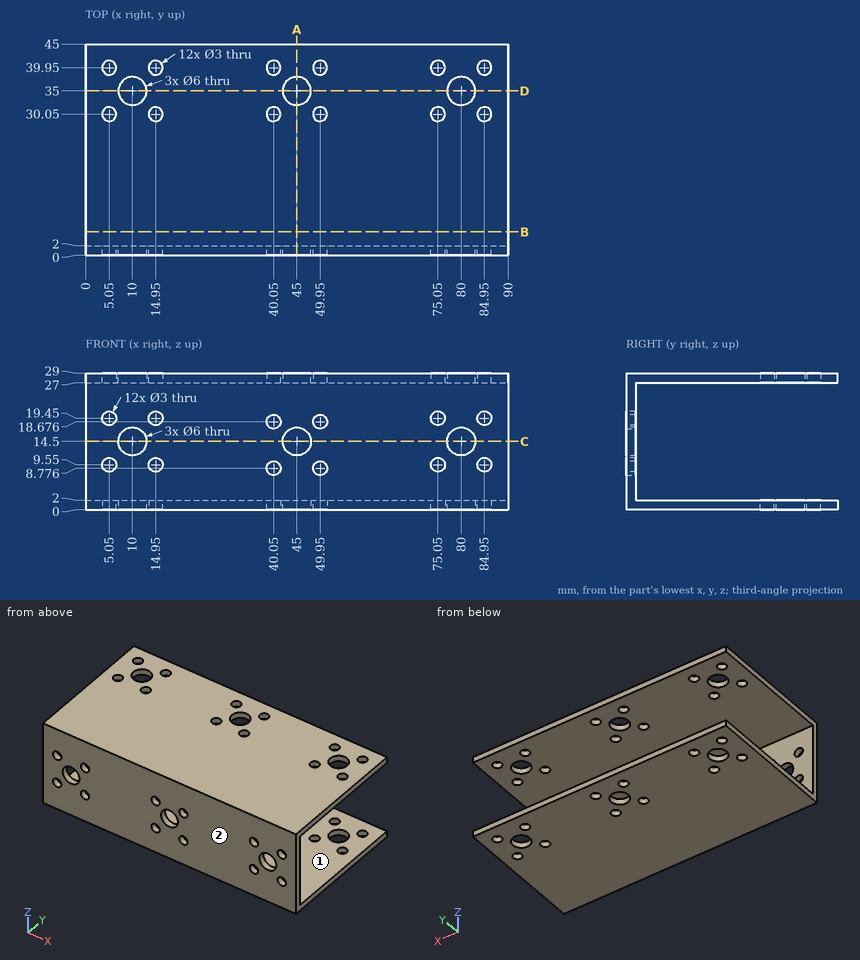
Study the drawing (mm; zero at the part's minimum x, y, z) and answer. A direction names the side the tool comes from. Round coordinates to 2 decimals unless told otherwise and drop trailing zeros. Loops run counter-clockwise (first coordinate to the right, second up) from the corner with the lowest first, then second, coordinate; pieces in that order, holes last. Notation, with made-up numbers: (28, 61.5) -> (77, 61.5) arc R20 cw to (77, 83.5) -> close; hole circle Ø2 at (-14, 40.5). An arc over 180 degrees is marked (long way). Use one line per item in the form item = value.
1. The part is cut by section D-D on y = 35. Give the number of separate pieces and of enclosed holes in the cut face, and give its area (3 significant figures).
Answer key:
separate_pieces = 8
enclosed_holes = 0
area = 288 mm²
2. Flat-ended cylindrical pins translate along their axes: pin 1 Ø2.5 at (x, y) = (40.05, 30.05) entering from -Z; pin 2 Ø5 at (x, z) = (15, 6.5) entering from +Y. Find the tip coordinate at first contact, or state that the pin passes through.
Answer key:
pin_1 = through
pin_2 = 2
3. A tool of negligible diameter and unlimited length cuts with its end or side. For the marked faces 1 and 2, from which of +Z, -Z, +X, -X, +Y, -Y can it reach the whole face along a straight path? Write none if from no direction.
Answer key:
face_1 = +X, -X, +Y
face_2 = +Z, -Z, +X, -X, -Y
4. The part is cut by section C-C on z = 14.5. Determine the outline of the cut face in (x, y), and give its area (3 significant figures).
Answer key:
outline = (0, 0) -> (7, 0) -> (7, 2) -> (0, 2) -> close; (13, 0) -> (42, 0) -> (42, 2) -> (13, 2) -> close; (48, 0) -> (77, 0) -> (77, 2) -> (48, 2) -> close; (83, 0) -> (90, 0) -> (90, 2) -> (83, 2) -> close
area = 144 mm²
5. The part is cut by section B-B on y = 5. Determine the outline of the cut face in (x, z).
Answer key:
outline = (0, 0) -> (90, 0) -> (90, 2) -> (0, 2) -> close; (0, 27) -> (90, 27) -> (90, 29) -> (0, 29) -> close
6. Find the intervals of material crossed by probe 1 along Z at (x, y) = (20, 7); probe 2 along X at (y, z) = (0.6, 14.5); probe 3 along Y at (x, z) = (37, 20), in increasing order. Write a range as [from, to].
Answer key:
probe_1 = [0, 2], [27, 29]
probe_2 = [0, 7], [13, 42], [48, 77], [83, 90]
probe_3 = [0, 2]
7. The part is cut by section A-A on x = 45. Determine the outline of the cut face in (y, z).
Answer key:
outline = (0, 0) -> (32, 0) -> (32, 2) -> (2, 2) -> (2, 11.5) -> (0, 11.5) -> close; (0, 17.5) -> (2, 17.5) -> (2, 27) -> (32, 27) -> (32, 29) -> (0, 29) -> close; (38, 0) -> (45, 0) -> (45, 2) -> (38, 2) -> close; (38, 27) -> (45, 27) -> (45, 29) -> (38, 29) -> close
